Can you work these out from the drawing? Everything is in mm from the part's minimum corner. A direction names the side the tool comes from. Round coordinates to 2 decimals unless told otherwise and drop trailing zeros. Write each loop counter-clockwise with the first axis right and the second up, starting at its lowest first coordinate (ties: lowest second). Pieces come first, ordered by that corner, then holes. Notation, with made-up numbers: (-3.5, 64.5) -> (0.5, 64.5) arc R34 ccw to (0.5, 103.5) -> close; hole circle Ø11 at (27.5, 75.25). An arc over 180 degrees is marked (long way). Answer as CSV lines item,"result".
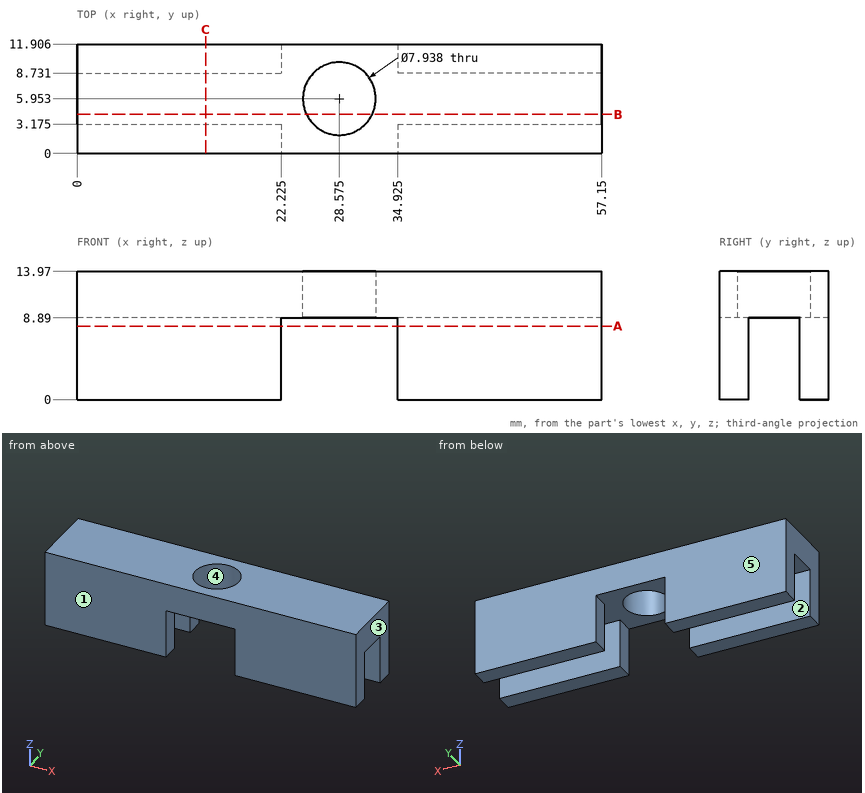
Item 1: Suppose I cut it at B-B, the plane y = 4.25. List the corners of the cut face in (x, z) for me, then the cut area to 3 significant figures.
Results found:
outline,"(0, 8.89) -> (24.99, 8.89) -> (24.99, 13.97) -> (0, 13.97) -> close; (32.16, 8.89) -> (57.15, 8.89) -> (57.15, 13.97) -> (32.16, 13.97) -> close"
area,"254 mm²"
Item 2: If we mould it in two halves opening along Y, with no side actions, what happens to the marked faces 3, 4 and 5? For each: pulls with the +Y half, pulls with the -Y half, needs draft (parallel to the pull), parting line crosses it, or undercut.
Results found:
face 3,"needs draft"
face 4,"undercut"
face 5,"pulls with the +Y half"
Item 3: Suppose I cut it at C-C, the plane x = 14. List the corners of the cut face in (y, z) for me (1 decimal).
Results found:
outline,"(0, 0) -> (3.2, 0) -> (3.2, 8.9) -> (8.7, 8.9) -> (8.7, 0) -> (11.9, 0) -> (11.9, 14) -> (0, 14) -> close"
Item 4: For the marked faces 1 and 2, which set-ups out of +Z, -Z, +X, -X, +Y, -Y let a thin tool reach every point of the face, with its end or its side?
Results found:
face 1,"+Z, -Z, +X, -X, -Y"
face 2,"-Z, +X, -X"
Item 5: I need wall thicknesses on L1, parallel to Y at x = 19.5, z = 1.5 (1 decimal); L2, parallel to Y at x = 28.5, z = 9.75 (1 decimal); L3, parallel to Z at x = 34.5, y = 10. Which ranges of each line are inside material? Lowest first, please.
Results found:
L1,"y = 0 to 3.2, 8.7 to 11.9"
L2,"y = 0 to 2, 9.9 to 11.9"
L3,"z = 8.89 to 13.97"
Item 6: Will these pins go through, and if not, where does the flat tip stop? pin 1 (3.5 mm diameter, centred on x = 35.5, y = 6, fed in from -Z); pin 2 (5 mm diameter, centred on x = 28.58, y = 5.95, fed in from -Z).
Results found:
pin 1,"stops at z = 8.89"
pin 2,"passes through"
Item 7: Suppose I cut it at A-A, the plane z = 8. State how many separate pieces and enclosed holes the cut face has, then the cut area to 3 significant figures.
Results found:
separate pieces,"4"
enclosed holes,"0"
area,"282 mm²"
